```python
from build123d import *

# Parameters (mm, degrees)
CYLINDER001_R     = 2.5
CYLINDER001_DEPTH = 13
BOX_W             = 12.25
BOX_H             = 23.78
BOX_DEPTH         = 22.68
BOX002_W          = 24.3
BOX002_H          = 21
BOX002_DEPTH      = 24
CYLINDER_R        = 2.5
CYLINDER_DEPTH    = 13


with BuildPart() as cylinder001:
    # Cylinder001 → Cylinder001 (new body)
    with BuildSketch(Plane(origin=(14.74, 17.5, -6.5), x_dir=(1, 0, 0), z_dir=(0, 0, 1))):
        Circle(CYLINDER001_R)
    extrude(amount=CYLINDER001_DEPTH)


with BuildPart() as servo:
    # Box → Box (new body)
    with BuildSketch(Plane(origin=(0, -1, 0), x_dir=(1, 0, 0), z_dir=(0, 0, 1))):
        with Locations((6.125, 11.89)):
            Rectangle(BOX_W, BOX_H)
    extrude(amount=BOX_DEPTH)


with BuildPart() as cut:
    # Box002 → Box002 (new body)
    with BuildSketch(Plane(origin=(-6, 0, 0), x_dir=(1, 0, 0), z_dir=(0, 0, 1))):
        with Locations((12.15, 10.5)):
            Rectangle(BOX002_W, BOX002_H)
    extrude(amount=BOX002_DEPTH)

    # Cut: cut servo
    add(servo.part, mode=Mode.SUBTRACT)


with BuildPart() as fusion:
    # Cylinder → Cylinder (new body)
    with BuildSketch(Plane(origin=(-2.5, 17.5, -6.5), x_dir=(1, 0, 0), z_dir=(0, 0, 1))):
        Circle(CYLINDER_R)
    extrude(amount=CYLINDER_DEPTH)

    # Fusion: union Cylinder001, Cut
    add(cylinder001.part)
    add(cut.part)


solid = fusion.part
```
Can you work these out from the model? Positions are in its coordinate system, mm. A direction names the side the tool comes from. Give positions to 0.01 mm unless a question says otherwise; leave off trailing zeros. Write each loop counter-clockwise with the first axis right and the second up, starting at its lowest first coordinate (ties: lowest second). Pieces come first, ordered by that corner, then holes. Notation, with made-up numbers: (80.5, 84) -> (91.5, 84) arc R28 ccw to (91.5, 120) -> close; hole circle Ø3 at (74.25, 56.5). An arc over 180 degrees is marked (long way). Write item = value, one per line.
(1) Thinking about a two-plate mould opening in X: for faces 1 (the face through (-2, 21, 12)), 2 (the face through (0, 10, 11)), 3 (the face through (6, 11, 22.68)), 4 (the face through (-6, 10, 12)), which applies, released by +X, released by -X, zero draft, split by the parting line, or undercut?
Worked out:
face_1 = zero draft
face_2 = undercut
face_3 = undercut
face_4 = released by -X
(2) Suppose I cut it at D-D on z = -2. Write out the boundary of the cut face in (x, y).
Worked out:
outline = circle Ø5 at (-2.5, 17.5); circle Ø5 at (14.74, 17.5)
(3) Suppose I cut it at A-A on z = 10.5. Write out the boundary of the cut face in (x, y), then the cut area to 3 significant figures.
Worked out:
outline = (-6, 0) -> (0, 0) -> (0, 21) -> (-6, 21) -> close; (12.25, 0) -> (18.3, 0) -> (18.3, 21) -> (12.25, 21) -> close
area = 253 mm^2
(4) Suppose I cut it at C-C on y = 11.25. Write out the boundary of the cut face in (x, z), then the cut area to 3 significant figures.
Worked out:
outline = (-6, 0) -> (0, 0) -> (0, 22.68) -> (12.25, 22.68) -> (12.25, 0) -> (18.3, 0) -> (18.3, 24) -> (-6, 24) -> close
area = 305 mm^2
(5) I'm going to push flat-ended pins straight in: P1, Ø10, axis at x = 6.5, y = 6, coming from the -Z side; P2, Ø5, axis at x = 1.5, y = 9, coming from the -Z side. Where does each tip first touch, or does it pass through?
Worked out:
P1 = 22.68
P2 = 0
(6) Suppose I cut it at B-B on x = -2.5. Write out the boundary of the cut face in (y, z), then the cut area to 4 significant figures.
Worked out:
outline = (0, 0) -> (15, 0) -> (15, -6.5) -> (20, -6.5) -> (20, 0) -> (21, 0) -> (21, 24) -> (0, 24) -> close
area = 536.5 mm^2
(7) For faces 5 (the face through (12.242, 17.61, -2.98)), 6 (the face through (6, 11, 24)), which set-ups out of +Z, -Z, +X, -X, +Y, -Y let a thin tool reach every point of the face, with its end or its side?
Worked out:
face_5 = -Z
face_6 = +Z, +X, -X, +Y, -Y
(8) I need wall thicknesses on probe 1 along X at (y, z) = (5.75, 15.5); probe 2 along Z at (x, y) = (4, 6); probe 3 along Z at (x, y) = (16, 14.25). Which ranges of each line are inside material? Lowest first, please. Write a range as from..to.
Worked out:
probe_1 = -6..0, 12.25..18.3
probe_2 = 22.68..24
probe_3 = 0..24
